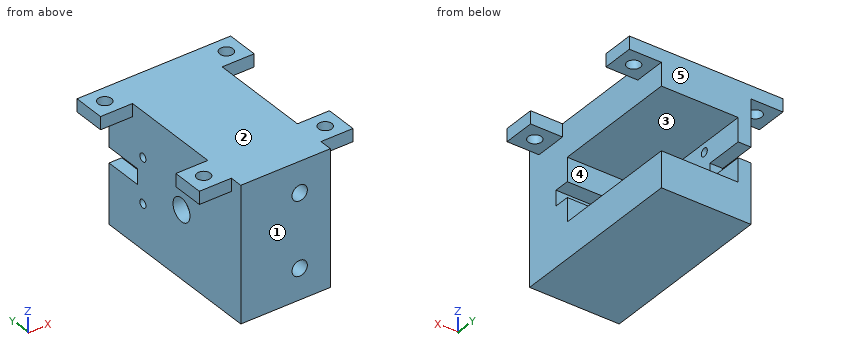
```python
from build123d import *

# Parameters (mm, degrees)
SKETCH1_W                = 40
SKETCH1_H                = 65
BOSS_EXTRUDE1_DEPTH      = 42.5
BOSS_EXTRUDE1_DEPTH_BACK = 15
SKETCH3_W                = 22.5
SKETCH3_H                = 50
CUT_EXTRUDE2_DEPTH       = 30
SKETCH4_R                = 4.5
CUT_EXTRUDE3_DEPTH       = 10
SKETCH6_W                = 40
SKETCH6_H                = 65
CUT_EXTRUDE4_DEPTH       = 5
SKETCH7_R                = 3
CUT_EXTRUDE5_DEPTH       = 10
SKETCH8_W                = 52.5
SKETCH8_H                = 65
CUT_EXTRUDE6_DEPTH       = 5
SKETCH9_W                = 12.5
SKETCH9_H                = 12.5
SKETCH9_R                = 2.6
BOSS_EXTRUDE2_DEPTH      = 5
SKETCH10_R               = 3
BOSS_EXTRUDE3_DEPTH      = 5
SKETCH11_R               = 1.6
CUT_EXTRUDE7_DEPTH       = 18.5
SKETCH12_W               = 30
SKETCH12_H               = 50
CUT_EXTRUDE8_DEPTH       = 12.25
CUT_EXTRUDE8_DEPTH_BACK  = 12.25
CUT_EXTRUDE9_DEPTH       = 30
CUT_EXTRUDE10_DEPTH      = 15


with BuildPart() as part:
    # Sketch1 → Boss-Extrude1 (new body, two sides)
    with BuildSketch(Plane.XY) as boss_extrude1_sk:
        with Locations((20, 32.5)):
            Rectangle(SKETCH1_W, SKETCH1_H)
    extrude(amount=BOSS_EXTRUDE1_DEPTH)
    extrude(boss_extrude1_sk.sketch, amount=-BOSS_EXTRUDE1_DEPTH_BACK)

    # Sketch3 → Cut-Extrude2 (cut)
    with BuildSketch(Plane(origin=(40, 0, 0), x_dir=(0, 0, -1), z_dir=(1, 0, 0))):
        with Locations((-11.25, 40)):
            Rectangle(SKETCH3_W, SKETCH3_H)
    extrude(amount=-CUT_EXTRUDE2_DEPTH, mode=Mode.SUBTRACT)

    # Sketch4 → Cut-Extrude3 (cut)
    with BuildSketch(Plane(origin=(10, 0, 0), x_dir=(0, 0, -1), z_dir=(1, 0, 0))):
        with Locations((-11.25, 26.5)):
            Circle(SKETCH4_R)
    extrude(amount=-CUT_EXTRUDE3_DEPTH, mode=Mode.SUBTRACT)

    # Sketch6 → Cut-Extrude4 (cut)
    with BuildSketch(Plane.XY.offset(42.5)):
        with Locations((20, 32.5)):
            Rectangle(SKETCH6_W, SKETCH6_H)
    extrude(amount=-CUT_EXTRUDE4_DEPTH, mode=Mode.SUBTRACT)

    # Sketch7 → Cut-Extrude5 (cut)
    with BuildSketch(Plane.XZ):
        with Locations((28, 25.5)):
            Circle(SKETCH7_R)
        with Locations((28, -3)):
            Circle(SKETCH7_R)
    extrude(amount=-CUT_EXTRUDE5_DEPTH, mode=Mode.SUBTRACT)

    # Sketch8 → Cut-Extrude6 (cut)
    with BuildSketch(Plane.ZY):
        with Locations((11.25, 32.5)):
            Rectangle(SKETCH8_W, SKETCH8_H)
    extrude(amount=-CUT_EXTRUDE6_DEPTH, mode=Mode.SUBTRACT)

    # Sketch9 → Boss-Extrude2 (add)
    with BuildSketch(Plane.XY.offset(37.5)):
        with Locations((-1.25, 58.75)):
            Rectangle(SKETCH9_W, SKETCH9_H)
        with Locations((-1.25, 58.75)):
            Circle(SKETCH9_R, mode=Mode.SUBTRACT)
        with Locations((46.25, 58.75)):
            Rectangle(SKETCH9_W, SKETCH9_H)
        with Locations((46.25, 58.75)):
            Circle(SKETCH9_R, mode=Mode.SUBTRACT)
        with Locations((46.25, 6.25)):
            Rectangle(SKETCH9_W, SKETCH9_H)
        with Locations((46.25, 6.25)):
            Circle(SKETCH9_R, mode=Mode.SUBTRACT)
        with Locations((-1.25, 6.25)):
            Rectangle(SKETCH9_W, SKETCH9_H)
        with Locations((-1.25, 6.25)):
            Circle(SKETCH9_R, mode=Mode.SUBTRACT)
    extrude(amount=-BOSS_EXTRUDE2_DEPTH)

    # Sketch10 → Boss-Extrude3 (add)
    with BuildSketch(Plane.XZ):
        Polygon((40, 32.5), (40, 37.5), (5, 37.5), (5, -15), (40, -15), align=None)
        with Locations((28, 25.5)):
            Circle(SKETCH10_R, mode=Mode.SUBTRACT)
        with Locations((28, -3)):
            Circle(SKETCH10_R, mode=Mode.SUBTRACT)
    extrude(amount=BOSS_EXTRUDE3_DEPTH)

    # Sketch11 → Cut-Extrude7 (cut, through all)
    with BuildSketch(Plane(origin=(10, 0, 0), x_dir=(0, 0, -1), z_dir=(1, 0, 0))):
        with Locations((-2.5, 47)):
            Circle(SKETCH11_R)
        with Locations((-20, 47)):
            Circle(SKETCH11_R)
    extrude(amount=-CUT_EXTRUDE7_DEPTH, mode=Mode.SUBTRACT)

    # Sketch12 → Cut-Extrude8 (cut, two sides)
    with BuildSketch(Plane(origin=(0, 0, 11.25), x_dir=(-1, 0, 0), z_dir=(0, 0, -1))) as cut_extrude8_sk:
        with Locations((-25, 40)):
            Rectangle(SKETCH12_W, SKETCH12_H)
    extrude(amount=CUT_EXTRUDE8_DEPTH, mode=Mode.SUBTRACT)
    extrude(cut_extrude8_sk.sketch, amount=-CUT_EXTRUDE8_DEPTH_BACK, mode=Mode.SUBTRACT)

    # Sketch13 → Cut-Extrude9 (cut)
    with BuildSketch(Plane(origin=(40, 0, 0), x_dir=(0, 0, -1), z_dir=(1, 0, 0))):
        Polygon((-11.25, 15), (-8.25, 15), (-8.25, 9), (-14.25, 9), (-14.25, 15), align=None)
    extrude(amount=-CUT_EXTRUDE9_DEPTH, mode=Mode.SUBTRACT)

    # Sketch14 → Cut-Extrude10 (cut)
    with BuildSketch(Plane(origin=(0, 65, 0), x_dir=(1, 0, 0), z_dir=(0, 1, 0))):
        Polygon((5, -11.25), (5, -8.25), (10, -8.25), (10, -14.25), (5, -14.25), align=None)
    extrude(amount=-CUT_EXTRUDE10_DEPTH, mode=Mode.SUBTRACT)


solid = part.part
```
CAD build for the part. Positions are in the model's coordinates, mm. Face numbers are marked on the shaded views. A direction names the side the tool comes from. Give positions to 0.01 mm unless a question says otherwise; leave off trailing zeros. Write each loop counter-clockwise with the first axis right and the second up, starting at its lowest first coordinate (ties: lowest second). Pieces come first, ordered by that corner, then holes. Notation, with made-up numbers: M 19,74 L 69,74 A19 cw 69,85 Z; hole C -13.5,76.5 d5. An arc over 180 degrees is marked long. Return JSON: item names as keys, results as strings. Group by question number.
(1) Band-saw the part on D-D (x = 11). Give the cut face in (y, z).
(2) Band-saw the part on C-C (x = 42). Give the cut face in (y, z).
(3) Drill centre lines: L1, parallel to Z at x = 28, y = 3.25; L2, parallel to Y at x = 46.25, z = 36.4; L3, parallel to Z at x = 29, y = 41. Where is each one in solid material? Low to high. Write a range as [from, to].
(4) Band-saw the part on B-B (z = 20). Give the cut face in (x, y), and give its area (3 significant figures).
(5) 3-axis set-ups, long thin cutter, end or side, ignore diameter. For the marked faces 4 and 5: which of +Z, -Z, +X, -X, +Y, -Y reach the whole face in a straight line?
(6) Flat gauge pins, fed straight in: pin 1 Ø11.5 at (y, z) = (26.5, 11.25) entering from +X; pin 2 Ø1.5 at (x, z) = (-3.5, 35) entering from -Y; pin 3 Ø4.5 at (x, z) = (22, 1.5) entering from +Y; pin 4 Ø4.5 at (x, y) = (46.25, 58.75) entering from -Z. Where does each tip first touch, or does it go through?
(7) Band-saw the part on A-A (y = 6.25). Give the cut face in (x, z).
(8) Mould opens along Z. For the marked faces 1, 2 and 3 say: pulls with the +Z half, pulls with the -Z half, needs draft (parallel to the pull), parting line crosses it, or undercut.
Entries:
{
 "1": {"outline": "M -5,-15 L 65,-15 L 65,-1 L 15,-1 L 15,8.25 L 9,8.25 L 9,14.25 L 15,14.25 L 15,23.5 L 65,23.5 L 65,37.5 L -5,37.5 Z"},
 "2": {"outline": "M 0,32.5 L 12.5,32.5 L 12.5,37.5 L 0,37.5 Z; M 52.5,32.5 L 65,32.5 L 65,37.5 L 52.5,37.5 Z"},
 "3": {"L1": "z = [-15, -6], [0, 22.5], [28.5, 37.5]", "L2": "y = [0, 3.65], [8.85, 12.5], [52.5, 56.15], [61.35, 65]", "L3": "z = [-15, -1], [23.5, 37.5]"},
 "4": {"outline": "M 5,-5 L 40,-5 L 40,15 L 10,15 L 10,45.4 L 5,45.4 Z; M 5,48.6 L 10,48.6 L 10,65 L 5,65 Z", "area": "934 mm^2"},
 "5": {"face 4": "+X, +Y", "face 5": "+Z, -Z, +X, -X, +Y"},
 "6": {"pin 1": "stops at x = 10", "pin 2": "stops at y = 0", "pin 3": "stops at y = 15", "pin 4": "passes through"},
 "7": {"outline": "M -7.5,32.5 L -3.85,32.5 L -3.85,37.5 L -7.5,37.5 Z; M 1.35,32.5 L 5,32.5 L 5,-15 L 40,-15 L 40,32.5 L 43.65,32.5 L 43.65,37.5 L 1.35,37.5 Z; M 48.85,32.5 L 52.5,32.5 L 52.5,37.5 L 48.85,37.5 Z; hole C 28,-3 d6; hole C 28,25.5 d6"},
 "8": {"face 1": "needs draft", "face 2": "pulls with the +Z half", "face 3": "undercut"}
}
